The figure shows three views and two pictorial views of one solid part (mm, origin at its lowest corner). Answer the questions. Give positions to 0.01 mm unless a question says otherwise; leave off trailing zeros. Loops run counter-clockwise (first coordinate to the right, second up) from the corner with the lowest first, then second, coordinate; pieces in that order, holes last. Notation, with made-up numbers: (78.5, -6.5) - (108.5, -6.5) arc R33 ccw to (108.5, 22.5) - close; hole circle Ø11 at (-34.75, -35.5). An arc over 180 degrees is marked (long way). Write item = value, one per line.
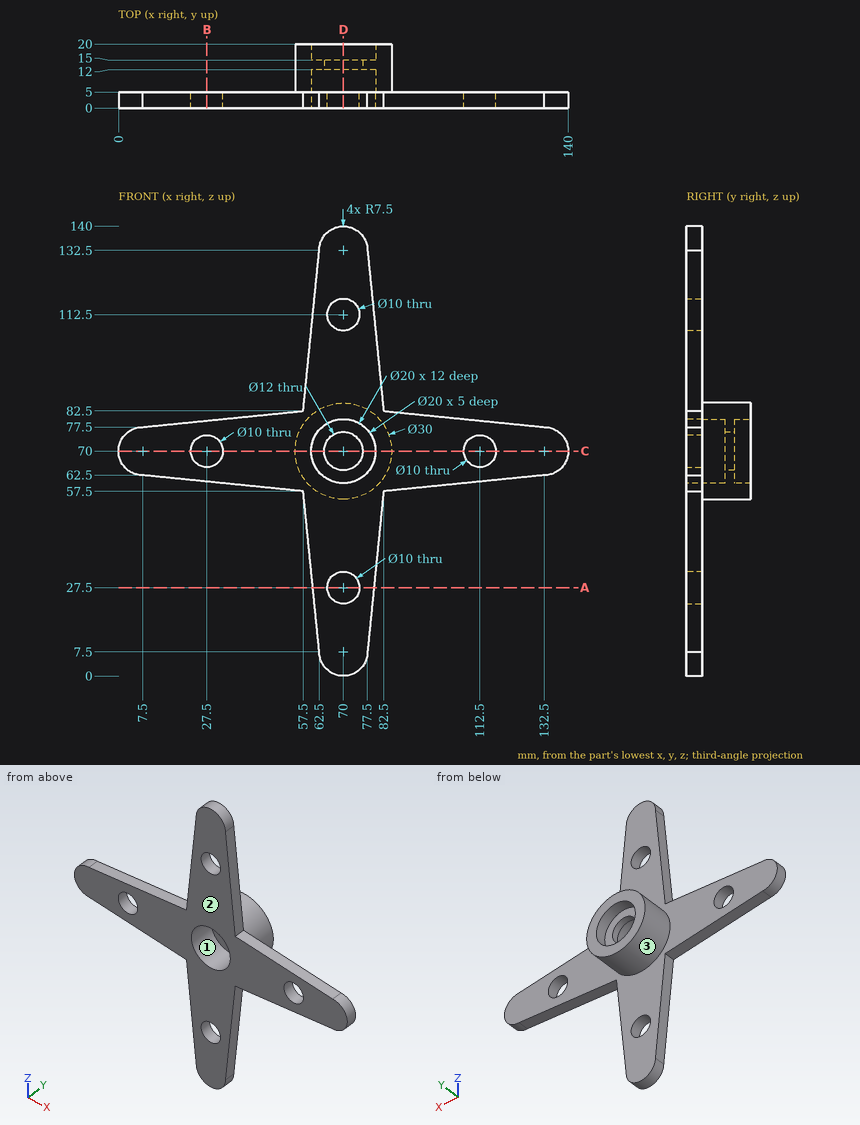
1) Each of these flat-tipped pins is pushed along its axis until it touches: P1, Ø16, axis at x = 70, z = 70, coming from the -Y side; P2, Ø3, axis at y = 2, z = 124.5, coming from the +X side; P3, Ø8, axis at x = 34, y = 2.5, coming from the -Z side; P4, Ø22, axis at x = 74, z = 67, coming from the -Y side. Where does it stop, or does it pass through?
Output:
P1 = 12
P2 = 78.45
P3 = 59.45
P4 = 0
2) A cutting plane is placed at C-C on z = 70. Determine the outline of the cut face in (x, y), then the cut area to 3 significant figures.
Output:
outline = (0, 0) - (22.5, 0) - (22.5, 5) - (0, 5) - close; (32.5, 0) - (60, 0) - (60, 12) - (64, 12) - (64, 15) - (60, 15) - (60, 20) - (55, 20) - (55, 5) - (32.5, 5) - close; (76, 12) - (80, 12) - (80, 0) - (107.5, 0) - (107.5, 5) - (85, 5) - (85, 20) - (80, 20) - (80, 15) - (76, 15) - close; (117.5, 0) - (140, 0) - (140, 5) - (117.5, 5) - close
area = 674 mm²
3) A cutting plane is placed at B-B on x = 27.5. Determine the outline of the cut face in (y, z).
Output:
outline = (0, 60.5) - (5, 60.5) - (5, 65) - (0, 65) - close; (0, 75) - (5, 75) - (5, 79.5) - (0, 79.5) - close
4) The mould has two halves that part along X. Classify the marked faces 1, 2 and 3: pulls with the +X half, pulls with the -X half, needs draft (parallel to the pull), parting line crosses it, or undercut.
Output:
face_1 = undercut
face_2 = needs draft
face_3 = parting line crosses it
5) A cutting plane is placed at D-D on x = 70. Determine the outline of the cut face in (y, z).
Output:
outline = (0, 0) - (5, 0) - (5, 22.5) - (0, 22.5) - close; (0, 32.5) - (5, 32.5) - (5, 55) - (20, 55) - (20, 60) - (15, 60) - (15, 64) - (12, 64) - (12, 60) - (0, 60) - close; (0, 80) - (12, 80) - (12, 76) - (15, 76) - (15, 80) - (20, 80) - (20, 85) - (5, 85) - (5, 107.5) - (0, 107.5) - close; (0, 117.5) - (5, 117.5) - (5, 140) - (0, 140) - close
6) Find the intervals of material crossed by probe 1 along X at (y, z) = (17.6, 70); probe 2 along X at (y, z) = (3.6, 27.5); probe 3 along Y at (x, z) = (64, 119), in increasing order.
Output:
probe_1 = 55 to 60, 80 to 85
probe_2 = 60.5 to 65, 75 to 79.5
probe_3 = 0 to 5
7) A cutting plane is placed at A-A on z = 27.5. Determine the outline of the cut face in (x, y).
Output:
outline = (60.5, 0) - (65, 0) - (65, 5) - (60.5, 5) - close; (75, 0) - (79.5, 0) - (79.5, 5) - (75, 5) - close
